Could you check a few things on this model? Use its own coordinates, in mm. Face numbers are marked on the shaded views. A direction names the side the tool comes from. Give positions to 0.01 mm unless a question says otherwise; leave off trailing zeros. Loops run counter-clockwise (first coordinate to the right, second up) from the corner with the lowest first, then second, coordinate; pieces in that order, holes last. Notation, with made-up numbers: (-10.5, 24) - (24.5, 24) arc R19 cw to (24.5, 45) - close; hole circle Ø9 at (46.25, 57.5). An arc over 180 degrees is marked (long way). Write each question's results on one line, items separated by ' | '. Start each with the question number.
Autodesk Inventor part; units mm, degrees
ref_plane "YZ Plane" through (0, 0, 0) normal (1, 0, 0) x (0, 1, 0)
ref_plane "XZ Plane" through (0, 0, 0) normal (0, 1, 0) x (-1, 0, 0)
ref_plane "XY Plane" through (0, 0, 0) normal (0, 0, 1) x (1, 0, 0)
sketch "Sketch1" plane through (0, 0, 0) normal (0, 1, 0) x (-1, 0, 0)
  circle A0 centre (0, 0) radius 7
  dimension "d0" = 14
extrude "Extrusion1" add sketch "Sketch1" along normal blind 15
sketch "Sketch2" plane through (0, 15, 0) normal (0, 1, 0) x (1, 0, 0)
  circle A0 centre (2.9736, 0) radius 2.141
  point P0 (0, 0)
extrude "Extrusion2" cut sketch "Sketch2" against normal blind 10
sketch "Sketch3" plane through (0, 0, 0) normal (0, -1, 0) x (1, 0, 0)
  circle A0 centre (0, 3.8062) radius 0.8659
  circle A1 centre (2.9736, -3.1401) radius 1.2343
  circle A2 centre (-2.7357, -2.141) radius 0.6471
  point P0 (0, 0)
extrude "Extrusion3" add sketch "Sketch3" along normal blind 5
properties part number "Conector de carga"
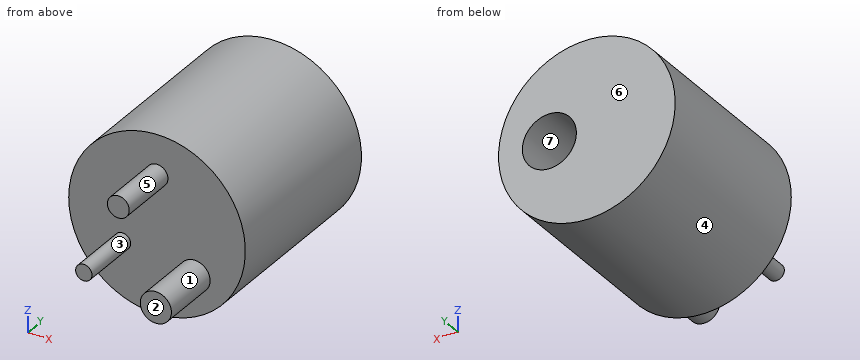
Q1. I need wall thicknesses on L1, parallel to Y at x = 3.5, z = 5.75; L2, parallel to Y at x = 2.75, z = 0.5; L3, parallel to Z at x = 4.25, y = 13.25. Which ranges of each line are inside material? Lowest first, please. Write a range as from..to.
Q2. I'm going to push flat-ended pins straight in: pin 1 Ø6 at (x, z) = (1, 0.5) entering from +Y; pin 2 Ø5 at (y, z) = (5.5, -5) entering from -X; pin 3 Ø4 at (y, z) = (9, -5) entering from -X; pin 4 Ø3.5 at (x, z) = (2.97, 0) entering from -Y. Where does each tip first touch, or does it pass through?
Q3. I want a section at D-D, the plane y = 2. List the corners of the cut face in (x, z) for me.
Q4. If we mould it in two halves opening along X, with no side actions, what happens to the marked faces 1, 2, 3 and 4? For each: +X half, -X half, draft (parallel to the pull), parting line (faces both ways), or undercut.
Q5. I want a section at C-C, the plane x = 0. List the corners of the cut face in (y, z) for me.
Q6. Which directions (+Z, -Z, +X, -X, +Y, -Y) give clear straight access to the entire face, cutting with the end or side of a thin tool? Please do the marked faces 5, 6 and 7.
Q7. I want a section at B-B, the plane y = 12. List the corners of the cut face in (x, z) for me, then the cut area to 3 significant figures.
Q8. I want a section at A-A, the plane z = 0. List the corners of the cut face in (x, y) for me.
Conclusion:
1) L1: 0..15 | L2: 0..5 | L3: -5.56..-1.72, 1.72..5.56
2) pin 1: y = 15 | pin 2: x = -6.54 | pin 3: x = -6.32 | pin 4: y = 0
3) outline: circle Ø14 at (0, 0)
4) face 1: undercut | face 2: draft | face 3: undercut | face 4: parting line
5) outline: (-5, 2.94) - (0, 2.94) - (0, -7) - (15, -7) - (15, 7) - (0, 7) - (0, 4.67) - (-5, 4.67) - close
6) face 5: -Y | face 6: +Z, -Z, +X, -X, +Y | face 7: +Y
7) outline: circle Ø14 at (0, 0); hole circle Ø4.28 at (2.97, 0) | area: 140 mm^2
8) outline: (-7, 0) - (7, 0) - (7, 15) - (5.11, 15) - (5.11, 5) - (0.83, 5) - (0.83, 15) - (-7, 15) - close
